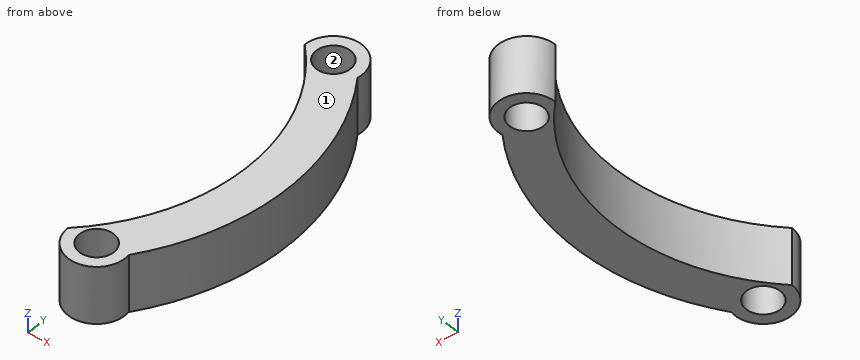
Autodesk Inventor part; units mm, degrees
ref_plane "YZ Plane" through (0, 0, 0) normal (1, 0, 0) x (0, 1, 0)
ref_plane "XZ Plane" through (0, 0, 0) normal (0, 1, 0) x (-1, 0, 0)
ref_plane "XY Plane" through (0, 0, 0) normal (0, 0, 1) x (1, 0, 0)
sketch "Sketch1" plane through (0, 0, 0) normal (0, 0, 1) x (1, 0, 0)
  circle A0 centre (0, 0) radius 1.5
  circle A1 centre (0, 25) radius 1.5
  arc A2 (2.4636, 24.5748) -> (0, 22.5) centre (0, 25) ccw
  arc A3 (-2.5, 0) -> (-0.4252, 2.4636) centre (0, 0) ccw
  line L0 (0, 16.5) -> (0, 25)
  arc A4 (0, -2.5) -> (0, 27.5) centre (-14.8423, 12.5) ccw
  arc A5 (-2.5, 0) -> (-2.5, 25) centre (-14.8423, 12.5) ccw
  dimension "d0" = 3
  dimension "d3" = 25
  dimension "d4" = 3
  dimension "d5" = 5
  dimension "d6" = 5
extrude "Extrusion1" add sketch "Sketch1" along normal blind 5 contours A4 A2 | A4 A3 A5 L0 A2 | A4 A3 A5 | A3 A4 | A2 L0 A5
properties part number "bar_mid"
Can you work these out from the model? Positions are in its coordinate system, mm. Face numbers are marked on the shaded views. Coordinates: 2 decimals unless noted, no trailing zeros. Loops run counter-clockwise (first coordinate to the right, second up) from the corner with the lowest first, then second, coordinate; pieces in that order, holes last. Notation, with made-up numbers: (45.25, 24) - (52.25, 24) arc R12 cw to (52.25, 43) - close; hole circle Ø8 at (15, 40.5). An arc over 180 degrees is marked (long way). Answer as CSV lines item,"result". Start each with the question number.
1) For pin 1 (2.5 mm diameter, centred on x = 0, y = 0, fed in from -Z); pin 2 (3 mm diameter, centred on y = 2, z = 4, fed in from +X); pin 3 (1.5 mm diameter, centred on y = 16.5, z = 2.5, fed in from +X); pin 4 (3 mm diameter, centred on y = 19, z = 3.5, fed in from -X), each with a flat end and sliding along its axis, tell me the tip position at first contact or that it passes through.
2) Suppose I cut it at C-C (y = 5). Please give me the cut outline in (x, z), plus the area to 3 significant figures.
3) Suppose I cut it at B-B (x = 0). Please give me the cut outline in (y, z).
4) Suppose I cut it at A-A (z = 0.4). Please give me the cut outline in (x, y), plus the area to 3 significant figures.
5) Thinking about a two-plate mould opening in Y: for the marked faces 1 and 2, which applies, pulls with the +Y half, pulls with the -Y half, needs draft (parallel to the pull), parting line crosses it, or undercut?
6) I need wall thicknesses on line 1 (Y direction, x = 0, z = 1.9); line 2 (Y direction, x = 1, z = 2); line 3 (X direction, y = 20, z = 1.2). Which ranges of each line are inside material? Lowest first, please. Write a range as from..to.
7) Suppose I cut it at D-D (x = 5.5). Please give me the cut outline in (y, z), plus the area to 3 significant figures.
Check result:
1,pin 1,"passes through"
1,pin 2,"stops at x = 4.24"
1,pin 3,"stops at x = 6.01"
1,pin 4,"stops at x = 0.8"
2,outline,"(1.04, 0) - (4.88, 0) - (4.88, 5) - (1.04, 5) - close"
2,area,"19.2 mm²"
3,outline,"(-2.5, 0) - (-1.5, 0) - (-1.5, 5) - (-2.5, 5) - close; (1.5, 0) - (3.1, 0) - (3.1, 5) - (1.5, 5) - close; (21.9, 0) - (23.5, 0) - (23.5, 5) - (21.9, 5) - close; (26.5, 0) - (27.5, 0) - (27.5, 5) - (26.5, 5) - close"
4,outline,"(-2.5, 0) arc R2.5 ccw (long way) to (2.46, 0.43) arc R21.1 ccw to (2.46, 24.57) arc R2.5 ccw (long way) to (-2.5, 25) arc R17.57 cw to start; hole circle Ø3 at (0, 0); hole circle Ø3 at (0, 25)"
4,area,"102 mm²"
5,face 1,"needs draft"
5,face 2,"undercut"
6,line 1,"y = -2.5..-1.5, 1.5..3.1, 21.9..23.5, 26.5..27.5"
6,line 2,"y = -2.29..-1.12, 1.12..4.91, 20.09..23.88, 26.12..27.29"
6,line 3,"x = 1.04..4.88"
7,outline,"(6.89, 0) - (18.11, 0) - (18.11, 5) - (6.89, 5) - close"
7,area,"56.1 mm²"
